```python
from build123d import *

# Parameters (mm, degrees)
SKETCH1_R           = 5
BOSS_EXTRUDE1_DEPTH = 2
SKETCH2_R           = 12
BOSS_EXTRUDE2_DEPTH = 2
SKETCH3_R           = 1.25
CUT_EXTRUDE1_DEPTH  = 18.435595774
CUT_EXTRUDE2_DEPTH  = 3
CUT_EXTRUDE3_START  = -1
SKETCH5_R           = 12
SKETCH5_R_2         = 3
CUT_EXTRUDE3_DEPTH  = 1
SKETCH6_R           = 2.5
CUT_EXTRUDE4_DEPTH  = 0.5
SKETCH7_R           = 0.5
CUT_EXTRUDE5_DEPTH  = 18.088007491


with BuildPart() as part:
    # Sketch1 → Boss-Extrude1 (new body)
    with BuildSketch(Plane(origin=(0, 0, 0), x_dir=(1, 0, 0), z_dir=(0, 1, 0))):
        with Locations(Location((0, 0, 0), (0, 0, 270))):
            Circle(SKETCH1_R)
    extrude(amount=BOSS_EXTRUDE1_DEPTH)

    # Sketch2 → Boss-Extrude2 (add)
    with BuildSketch(Plane(origin=(0, 2, 0), x_dir=(1, 0, 0), z_dir=(0, 1, 0))):
        with Locations(Location((0, 0, 0), (0, 0, 270))):
            Circle(SKETCH2_R)
    extrude(amount=BOSS_EXTRUDE2_DEPTH)

    # Sketch3 → Cut-Extrude1 (cut, through all)
    with BuildSketch(Plane.XZ):
        with Locations(Location((0, 0, 0), (0, 0, 270))):
            Circle(SKETCH3_R)
    extrude(amount=-CUT_EXTRUDE1_DEPTH, mode=Mode.SUBTRACT)

    # Sketch4 → Cut-Extrude2 (cut)
    with BuildSketch(Plane.XZ):
        with BuildLine():
            Line((0.25, 2.25), (0.25, 1.984313483))
            ThreePointArc((0.25, 1.984313483), (0.367499036, 1.965946199), (0.483698652, 1.940627634))
            Line((0.483698652, 1.940627634), (0.579675692, 2.188372933))
            ThreePointArc((0.579675692, 2.188372933), (0.903104165, 2.331180574), (1.045911806, 2.0077521))
            Line((1.045911806, 2.0077521), (0.949934766, 1.760006801))
            ThreePointArc((0.949934766, 1.760006801), (1.052864326, 1.700434271), (1.15207112, 1.63484927))
            Line((1.15207112, 1.63484927), (1.331062969, 1.831193975))
            ThreePointArc((1.331062969, 1.831193975), (1.684239109, 1.847522293), (1.700567428, 1.494346153))
            Line((1.700567428, 1.494346153), (1.521575579, 1.298001448))
            ThreePointArc((1.521575579, 1.298001448), (1.596034455, 1.205269273), (1.66485, 1.108275452))
            Line((1.66485, 1.108275452), (1.902682817, 1.226702123))
            ThreePointArc((1.902682817, 1.226702123), (2.237908228, 1.114345889), (2.125551994, 0.779120478))
            Line((2.125551994, 0.779120478), (1.887719178, 0.660693807))
            ThreePointArc((1.887719178, 0.660693807), (1.923651286, 0.54732598), (1.952781662, 0.432022894))
            Line((1.952781662, 0.432022894), (2.217334807, 0.456537353))
            ThreePointArc((2.217334807, 0.456537353), (2.489335441, 0.230670899), (2.263468987, -0.041329735))
            Line((2.263468987, -0.041329735), (1.998915842, -0.065844194))
            ThreePointArc((1.998915842, -0.065844194), (1.991468353, -0.184536719), (1.97697934, -0.30257675))
            Line((1.97697934, -0.30257675), (2.232523445, -0.375285317))
            ThreePointArc((2.232523445, -0.375285317), (2.404564108, -0.684157475), (2.09569195, -0.856198138))
            Line((2.09569195, -0.856198138), (1.840147845, -0.783489572))
            ThreePointArc((1.840147845, -0.783489572), (1.790326583, -0.891476712), (1.734175003, -0.996311728))
            Line((1.734175003, -0.996311728), (1.94619742, -1.156423625))
            ThreePointArc((1.94619742, -1.156423625), (1.995043068, -1.506586591), (1.644880102, -1.555432239))
            Line((1.644880102, -1.555432239), (1.432857685, -1.395320341))
            ThreePointArc((1.432857685, -1.395320341), (1.347391287, -1.478017834), (1.257160723, -1.555489285))
            Line((1.257160723, -1.555489285), (1.39702665, -1.781380515))
            ThreePointArc((1.39702665, -1.781380515), (1.316080407, -2.125542839), (0.971918083, -2.044596596))
            Line((0.971918083, -2.044596596), (0.832052155, -1.818705367))
            ThreePointArc((0.832052155, -1.818705367), (0.722483332, -1.864944459), (0.610359921, -1.904589396))
            Line((0.610359921, -1.904589396), (0.65917969, -2.165752095))
            ThreePointArc((0.65917969, -2.165752095), (0.459373795, -2.457432749), (0.16769314, -2.257626854))
            Line((0.16769314, -2.257626854), (0.118873371, -1.996464155))
            ThreePointArc((0.118873371, -1.996464155), (0, -2), (-0.118873371, -1.996464155))
            Line((-0.118873371, -1.996464155), (-0.16769314, -2.257626854))
            ThreePointArc((-0.16769314, -2.257626854), (-0.459373795, -2.457432749), (-0.65917969, -2.165752095))
            Line((-0.65917969, -2.165752095), (-0.610359921, -1.904589396))
            ThreePointArc((-0.610359921, -1.904589396), (-0.722483332, -1.864944459), (-0.832052155, -1.818705367))
            Line((-0.832052155, -1.818705367), (-0.971918083, -2.044596596))
            ThreePointArc((-0.971918083, -2.044596596), (-1.316080407, -2.125542839), (-1.39702665, -1.781380515))
            Line((-1.39702665, -1.781380515), (-1.257160723, -1.555489285))
            ThreePointArc((-1.257160723, -1.555489285), (-1.347391287, -1.478017834), (-1.432857685, -1.395320341))
            Line((-1.432857685, -1.395320341), (-1.644880102, -1.555432239))
            ThreePointArc((-1.644880102, -1.555432239), (-1.995043068, -1.506586591), (-1.94619742, -1.156423625))
            Line((-1.94619742, -1.156423625), (-1.734175003, -0.996311728))
            ThreePointArc((-1.734175003, -0.996311728), (-1.790326583, -0.891476712), (-1.840147845, -0.783489572))
            Line((-1.840147845, -0.783489572), (-2.09569195, -0.856198138))
            ThreePointArc((-2.09569195, -0.856198138), (-2.404564108, -0.684157475), (-2.232523445, -0.375285317))
            Line((-2.232523445, -0.375285317), (-1.97697934, -0.30257675))
            ThreePointArc((-1.97697934, -0.30257675), (-1.991468353, -0.184536719), (-1.998915842, -0.065844194))
            Line((-1.998915842, -0.065844194), (-2.263468987, -0.041329735))
            ThreePointArc((-2.263468987, -0.041329735), (-2.489335441, 0.230670899), (-2.217334807, 0.456537353))
            Line((-2.217334807, 0.456537353), (-1.952781662, 0.432022894))
            ThreePointArc((-1.952781662, 0.432022894), (-1.923651286, 0.54732598), (-1.887719178, 0.660693807))
            Line((-1.887719178, 0.660693807), (-2.125551994, 0.779120478))
            ThreePointArc((-2.125551994, 0.779120478), (-2.237908228, 1.114345889), (-1.902682817, 1.226702123))
            Line((-1.902682817, 1.226702123), (-1.66485, 1.108275452))
            ThreePointArc((-1.66485, 1.108275452), (-1.596034455, 1.205269273), (-1.521575579, 1.298001448))
            Line((-1.521575579, 1.298001448), (-1.700567428, 1.494346153))
            ThreePointArc((-1.700567428, 1.494346153), (-1.684239109, 1.847522293), (-1.331062969, 1.831193975))
            Line((-1.331062969, 1.831193975), (-1.15207112, 1.63484927))
            ThreePointArc((-1.15207112, 1.63484927), (-1.052864326, 1.700434271), (-0.949934766, 1.760006801))
            Line((-0.949934766, 1.760006801), (-1.045911806, 2.0077521))
            ThreePointArc((-1.045911806, 2.0077521), (-0.903104165, 2.331180574), (-0.579675692, 2.188372933))
            Line((-0.579675692, 2.188372933), (-0.483698652, 1.940627634))
            ThreePointArc((-0.483698652, 1.940627634), (-0.367499036, 1.965946199), (-0.25, 1.984313483))
            Line((-0.25, 1.984313483), (-0.25, 2.25))
            ThreePointArc((-0.25, 2.25), (0, 2.5), (0.25, 2.25))
        make_face()
    extrude(amount=-CUT_EXTRUDE2_DEPTH, mode=Mode.SUBTRACT)

    # Sketch5 → Cut-Extrude3 (cut)
    with BuildSketch(Plane(origin=(0, 4, 0), x_dir=(1, 0, 0), z_dir=(0, 1, 0)).offset(CUT_EXTRUDE3_START)):
        with Locations(Location((0, 0, 0), (0, 0, 270))):
            Circle(SKETCH5_R)
        with Locations(Location((0, 0, 0), (0, 0, 270))):
            Circle(SKETCH5_R_2, mode=Mode.SUBTRACT)
    extrude(amount=CUT_EXTRUDE3_DEPTH, mode=Mode.SUBTRACT)

    # Sketch6 → Cut-Extrude4 (cut)
    with BuildSketch(Plane(origin=(0, 4, 0), x_dir=(1, 0, 0), z_dir=(0, 1, 0))):
        with Locations(Location((0, 0, 0), (0, 0, 270))):
            Circle(SKETCH6_R)
    extrude(amount=-CUT_EXTRUDE4_DEPTH, mode=Mode.SUBTRACT)

    # Sketch7 → Cut-Extrude5 (cut, through all)
    with BuildSketch(Plane.XZ.offset(-2)):
        with Locations(Location((0, 8, 0), (0, 0, 270))):
            Circle(SKETCH7_R)
        with Locations(Location((2.5, 7.599342077, 0), (0, 0, 270))):
            Circle(SKETCH7_R)
        with Locations(Location((-2.5, 7.599342077, 0), (0, 0, 270))):
            Circle(SKETCH7_R)
        with Locations(Location((8, 0, 0), (0, 0, 270))):
            Circle(SKETCH7_R)
        with Locations(Location((7.599342077, -2.5, 0), (0, 0, 270))):
            Circle(SKETCH7_R)
        with Locations(Location((7.599342077, 2.5, 0), (0, 0, 270))):
            Circle(SKETCH7_R)
        with Locations(Location((0, -8, 0), (0, 0, 270))):
            Circle(SKETCH7_R)
        with Locations(Location((-2.5, -7.599342077, 0), (0, 0, 270))):
            Circle(SKETCH7_R)
        with Locations(Location((2.5, -7.599342077, 0), (0, 0, 270))):
            Circle(SKETCH7_R)
        with Locations(Location((-8, 0, 0), (0, 0, 270))):
            Circle(SKETCH7_R)
        with Locations(Location((-7.599342077, 2.5, 0), (0, 0, 270))):
            Circle(SKETCH7_R)
        with Locations(Location((-7.599342077, -2.5, 0), (0, 0, 270))):
            Circle(SKETCH7_R)
        with Locations(Location((10.099342077, 2.5, 0), (0, 0, 270))):
            Circle(SKETCH7_R)
        with Locations(Location((10.099342077, -2.5, 0), (0, 0, 270))):
            Circle(SKETCH7_R)
        with Locations(Location((10.5, 0, 0), (0, 0, 270))):
            Circle(SKETCH7_R)
        with Locations(Location((-10.099342077, 2.5, 0), (0, 0, 270))):
            Circle(SKETCH7_R)
        with Locations(Location((-10.099342077, -2.5, 0), (0, 0, 270))):
            Circle(SKETCH7_R)
        with Locations(Location((-10.5, 0, 0), (0, 0, 270))):
            Circle(SKETCH7_R)
    extrude(amount=-CUT_EXTRUDE5_DEPTH, mode=Mode.SUBTRACT)


solid = part.part
```
Work out the finished part from the listing and answer in its coordinate system (mm). A direction names the side the tool comes from. Coordinates: 2 decimals unless noted, no trailing zeros. Order: outer loops, then holes, each group sorted by start corner. A loop starts at its lowest first (then second) coordinate and runs counter-clockwise, first axis right, second up. Notation, with made-up numbers: M 88.25,30.25 L 118.25,30.25 A24 cw 118.25,66.25 Z; hole C 28,17 d7. An arc over 180 degrees is marked long. Use CSV: the item, a comma, the result in double quotes.
1) For faces 4 (the face through (-1, 3, 1)), 5 (the face through (1, 3.5, 1)), 6 (the face through (-0.192, 2.493, 7.538)), determine the directions among +Z, -Z, +X, -X, +Y, -Y from which every point of the face is accessible in a straight line to the end or side of a thin tool.
Worked out:
face 4,"-Y"
face 5,"+Y"
face 6,"+Y, -Y"
2) Consider line 1 (Y direction, x = -8, z = 5.5); line 2 (X direction, y = 2.3, z = 0); line 3 (X direction, y = 1.1, z = 2.25). Determine where each line is inside the solid, lowest interval first. Write a range as [from, to].
Worked out:
line 1,"y = [2, 3]"
line 2,"x = [-12, -11], [-10, -8.5], [-7.5, -2.38], [2.38, 7.5], [8.5, 10], [11, 12]"
line 3,"x = [-4.47, -1.01], [-0.61, -0.25], [0.25, 0.61], [1.01, 4.47]"
3) Section A-A on z = -4.5 is taken. Write down the section's boundary in (x, y).
Worked out:
outline,"M -11.12,2 L -2.18,2 L -2.18,0 L 2.18,0 L 2.18,2 L 11.12,2 L 11.12,3 L -11.12,3 Z"
4) Section B-B on y = 2.7 is taken. Count the separate pieces of the cut face and the enclosed holes in it, plus the area to 3 significant figures.
Worked out:
separate pieces,"1"
enclosed holes,"19"
area,"422 mm^2"
5) Flat-ended cylindrical pins translate along their axes: pin 1 Ø5.5 at (x, z) = (0.5, -1) entering from +Y; pin 2 Ø4.5 at (x, z) = (0, 0) entering from +Y; pin 3 Ø5 at (x, z) = (8.5, 5.5) entering from +Y. Find the tip coordinate at first contact, or state that the pin passes through.
Worked out:
pin 1,"stops at y = 4"
pin 2,"stops at y = 3.5"
pin 3,"stops at y = 3"
6) Section C-C on x = 6.25 is taken. Write down the section's boundary in (y, z).
Worked out:
outline,"M 2,-10.24 L 3,-10.24 L 3,10.24 L 2,10.24 Z"
7) Determine the mould class of faces 1 (the face through (2.5, 2.5, -7.1)), 2 (the face through (3.604, 2.493, 11.446)), 3 (the face through (3, 3, 2)) for opening direction Z: released by +Z, released by -Z, zero draft, split by the parting line, or undercut.
Worked out:
face 1,"undercut"
face 2,"split by the parting line"
face 3,"zero draft"
